from build123d import *

# Parameters (mm, degrees)
SKETCH2_W           = 120
SKETCH2_H           = 140
BOSS_EXTRUDE1_DEPTH = 50
SKETCH3_R           = 3
SKETCH3_W           = 80
SKETCH3_H           = 70
CUT_EXTRUDE1_DEPTH  = 47
CUT_EXTRUDE3_START  = -10
SKETCH4_W           = 80
SKETCH4_H           = 40
CUT_EXTRUDE3_DEPTH  = 37
SKETCH5_W           = 11
SKETCH5_H           = 12
CUT_EXTRUDE4_DEPTH  = 20


with BuildPart() as part:
    # Sketch2 → Boss-Extrude1 (new body)
    with BuildSketch(Plane.XY):
        with Locations((-60, -70)):
            Rectangle(SKETCH2_W, SKETCH2_H)
    extrude(amount=BOSS_EXTRUDE1_DEPTH)

    # Sketch3 → Cut-Extrude1 (cut)
    with BuildSketch(Plane.XY.offset(50)):
        with Locations((-110, -55)):
            Circle(SKETCH3_R)
        with Locations((-10, -55)):
            Circle(SKETCH3_R)
        with Locations((-60, -55)):
            Rectangle(SKETCH3_W, SKETCH3_H)
    extrude(amount=-CUT_EXTRUDE1_DEPTH, mode=Mode.SUBTRACT)

    # Sketch4 → Cut-Extrude3 (cut)
    with BuildSketch(Plane.XY.offset(50).offset(CUT_EXTRUDE3_START)):
        with Locations((-60, -110)):
            Rectangle(SKETCH4_W, SKETCH4_H)
    extrude(amount=-CUT_EXTRUDE3_DEPTH, mode=Mode.SUBTRACT)

    # Sketch5 → Cut-Extrude4 (cut)
    with BuildSketch(Plane(origin=(0, 0, 0), x_dir=(0, 0, -1), z_dir=(1, 0, 0))):
        with Locations((-8.5, -124)):
            Rectangle(SKETCH5_W, SKETCH5_H)
    extrude(amount=-CUT_EXTRUDE4_DEPTH, mode=Mode.SUBTRACT)


solid = part.part
Geometry: final body of the model. Coordinates: model frame, mm. A direction names the side the tool comes from. Coordinates: 2 decimals unless noted, no trailing zeros. Loops run counter-clockwise (first coordinate to the right, second up) from the corner with the lowest first, then second, coordinate; pieces in that order, holes last. Notation, with made-up numbers: (-29.75, 87.25) - (22.25, 87.25) arc R19 ccw to (22.25, 118.25) - close; hole circle Ø8 at (15.5, -28.5). An arc over 180 degrees is marked (long way). Put each result on its own line as item: value. Start each with the question number.
Q1. Pin query (flat end, axial travel): pin 1 Ø3 at (x, y) = (-109.5, -54.5) entering from +Z. Return the tip coordinate at first contact, or that it passes through.
Q2. Pull-direction query (Z, two-part tool) for faces 5 (the flat face through (-61, -90, 45)), 6 (the flat face through (-61, -69, 0)), 7 (the flat face through (-61, -110, 40)); classes: released by +Z, released by -Z, zero draft, split by the parting line, or undercut.
Q3. Cut plane D-D, the plane z = 45. Return loops of the section in (x, y), and give its area (3 significant figures).
Q4. Cut plane C-C, the plane y = -55. Return loops of the section in (x, z), and give its area (3 significant figures).
Q5. Line query: line 1 (Y direction, x = -10, z = 13.5); line 2 (Y direction, x = -97, z = 41); line 3 (Z direction, x = -47, y = -109.5). Output: solid intervals per line, ascending.
Q6. Cut plane B-B, the plane x = -10. Return loops of the section in (y, z), and give its area (3 significant figures).
Q7. Cut plane A-A, the plane z = 7. Return loops of the section in (x, y), and give its area (3 significant figures).
Q8. Set-up query: faces 1 (the flat face through (-61, -140, 25)), 2 (the cylindrical face through (-108.39, -52.47, 26.83)), 3 (the flat face through (-10, -118, 9)), 4 (the flat face through (-100, -76, 27)). Return all of +Z, -Z, +X, -X, +Y, -Y with unobstructed straight access to the full face (end or side cutting, diameter ignored); none if empty.
Filled sheet:
1. pin 1: z = 3
2. face 5: zero draft
2. face 6: released by -Z
2. face 7: undercut
3. outline: (-120, -140) - (0, -140) - (0, 0) - (-120, 0) - close; hole circle Ø6 at (-110, -55); hole (-100, -90) - (-20, -90) - (-20, -20) - (-100, -20) - close; hole circle Ø6 at (-10, -55)
3. area: 11,100 mm²
4. outline: (-120, 0) - (0, 0) - (0, 50) - (-7, 50) - (-7, 3) - (-13, 3) - (-13, 50) - (-20, 50) - (-20, 3) - (-100, 3) - (-100, 50) - (-107, 50) - (-107, 3) - (-113, 3) - (-113, 50) - (-120, 50) - close
4. area: 1,680 mm²
5. line 1: -140 to -130, -118 to -58, -52 to 0
5. line 2: -140 to -90, -20 to 0
5. line 3: 0 to 3, 40 to 50
6. outline: (-140, 0) - (0, 0) - (0, 50) - (-52, 50) - (-52, 3) - (-58, 3) - (-58, 50) - (-140, 50) - close; hole (-130, 3) - (-118, 3) - (-118, 14) - (-130, 14) - close
6. area: 6,590 mm²
7. outline: (-120, -140) - (0, -140) - (0, -130) - (-100, -130) - (-100, -20) - (-20, -20) - (-20, -118) - (0, -118) - (0, 0) - (-120, 0) - close; hole circle Ø6 at (-110, -55); hole circle Ø6 at (-10, -55)
7. area: 7,700 mm²
8. face 1: +Z, -Z, +X, -X, -Y
8. face 2: +Z
8. face 3: +X
8. face 4: none
